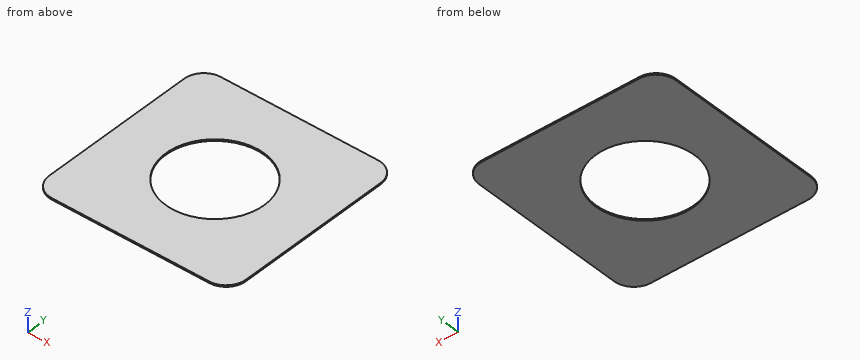
Autodesk Inventor part; units mm, degrees
ref_plane "YZ Plane" through (0, 0, 0) normal (1, 0, 0) x (0, 1, 0)
ref_plane "XZ Plane" through (0, 0, 0) normal (0, 1, 0) x (-1, 0, 0)
ref_plane "XY Plane" through (0, 0, 0) normal (0, 0, 1) x (1, 0, 0)
sketch "スケッチ1" plane through (0, 0, 0) normal (0, 0, 1) x (1, 0, 0)
  line L0 (-10, 10) -> (10, 10)
  line L1 (10, 10) -> (10, -10)
  line L2 (10, -10) -> (-10, -10)
  line L3 (-10, -10) -> (-10, 10)
  point P0 (0, 0)
  dimension "d0" = 10
  dimension "d1" = 20
  dimension "d2" = 10
  dimension "d3" = 20
extrude "押し出し1" add sketch "スケッチ1" along normal blind 0.16
sketch "スケッチ2" plane through (0, 0, 0) normal (0, 0, 1) x (1, 0, 0)
  circle A0 centre (0, 0) radius 5
  dimension "d6" = 10
extrude "押し出し2" cut sketch "スケッチ2" along normal blind 0.16
fillet "フィレット1" radius 2 4 edges at (10, 10, 0.08) (-10, 10, 0.08) (10, -10, 0.08) (-10, -10, 0.08)
properties part number "HbSensorTape01"
Part model, mm, in its own coordinate system. Give positions to 0.01 mm unless a question says otherwise; leave off trailing zeros. Loops run counter-clockwise (first coordinate to the right, second up) from the corner with the lowest first, then second, coordinate; pieces in that order, holes last. Notation, with made-up numbers: M 59.25,-39 L 89.25,-39 A31 cw 89.25,0 Z; hole C 47,63.5 d10. An arc over 180 degrees is marked long. Return JSON: item names as keys, results as strings.
1) Saw through at A-A, the plane x = 0. List the corners of the cut face in (y, z).
Calculated:
{"outline": "M -10,0 L -5,0 L -5,0.16 L -10,0.16 Z; M 5,0 L 10,0 L 10,0.16 L 5,0.16 Z"}
2) Drill centre lines: line 1 (Y direction, x = 0, z = 0.1); line 2 (Y direction, x = -1, z = 0.1); line 3 (Y direction, x = 8.25, z = 0.1). Where is each one in solid material? Low to high.
Calculated:
{"line 1": "y = -10 to -5, 5 to 10", "line 2": "y = -10 to -4.9, 4.9 to 10", "line 3": "y = -9.98 to 9.98"}
3) Saw through at B-B, the plane z = 0.1. List the corners of the cut face in (x, y).
Calculated:
{"outline": "M -10,-8 A2 ccw -8,-10 L 8,-10 A2 ccw 10,-8 L 10,8 A2 ccw 8,10 L -8,10 A2 ccw -10,8 Z; hole C 0,0 d10"}
